Autodesk Inventor part; units mm, degrees
ref_plane "YZ Plane" through (0, 0, 0) normal (1, 0, 0) x (0, 1, 0)
ref_plane "XZ Plane" through (0, 0, 0) normal (0, 1, 0) x (-1, 0, 0)
ref_plane "XY Plane" through (0, 0, 0) normal (0, 0, 1) x (1, 0, 0)
sketch "Szkic1" plane through (0, 0, 0) normal (0, 1, 0) x (-1, 0, 0)
  line L0 (0, 0) -> (-15, 0)
  line L1 (0, 0) -> (15, 0)
  circle A0 centre (0, 0) radius 5
  circle A1 centre (15, 0) radius 2
  circle A2 centre (-15, 0) radius 2
  line L2 (-19, 7.5) -> (19, 7.5)
  line L3 (19, 7.5) -> (19, -7.5)
  line L4 (19, -7.5) -> (-19, -7.5)
  line L5 (-19, -7.5) -> (-19, 7.5)
  line L6 (-19, 7.5) -> (19, -7.5) construction
  line L7 (19, 7.5) -> (-19, -7.5) construction
  line L8 (0, 0) -> (15, 0)
  line L9 (6, 2.5) -> (9, 2.5)
  line L10 (9, 2.5) -> (9, -2.5)
  line L11 (9, -2.5) -> (6, -2.5)
  line L12 (6, -2.5) -> (6, 2.5)
  line L13 (6, 2.5) -> (9, -2.5) construction
  line L14 (9, 2.5) -> (6, -2.5) construction
  line L15 (-9, 2.5) -> (-6, 2.5)
  line L16 (-6, 2.5) -> (-6, -2.5)
  line L17 (-6, -2.5) -> (-9, -2.5)
  line L18 (-9, -2.5) -> (-9, 2.5)
  line L19 (-9, 2.5) -> (-6, -2.5) construction
  line L20 (-6, 2.5) -> (-9, -2.5) construction
  point P0 (7.5, 0)
  point P1 (-7.5, 0)
  point P2 (-5, 0)
  point P3 (5, 0)
  dimension "d0" = 15
  dimension "d1" = 15
  dimension "d2" = 10
  dimension "d3" = 4
  dimension "d4" = 4
  dimension "d5" = 38
  dimension "d6" = 15
  dimension "d7" = 3
  dimension "d8" = 5
  dimension "d9" = 3
  dimension "d10" = 5
extrude "Wyciągnięcie proste1" add sketch "Szkic1" along normal blind 1 contours L16 L17 L18 L0 | L0 L18 L15 L16 | L12 L9 L10 L1 | L1 L10 L11 L12 | L2 L3 L4 L5
extrude "Wyciągnięcie proste2" add sketch "Szkic1" along normal blind 30 contours L16 L17 L18 L0 | L0 L18 L15 L16
sketch "Szkic2" plane through (-6, 1, -2.5) normal (1, 0, 0) x (0, 0, -1)
  line L0 (0, 19) -> (-5, 19)
  line L1 (0, 19) -> (-2.12132, 16.87868)
  line L2 (0, 19) -> (3, 19) construction
  circle A0 centre (-2.12132, 16.87868) radius 1.5
  point P0 (-2.5, -1)
  dimension "d15" = 3
  dimension "d16" = 135
  dimension "d17" = 3
extrude "Wyciągnięcie proste3" [suppressed]
fillet "Zaokrąglenie1" radius 1 4 edges at (6, 15.5, -2.5) (9, 15.5, -2.5) (9, 15.5, 2.5) (6, 15.5, 2.5)
sketch "Szkic3" plane through (6, 1, 1.5) normal (-1, 0, 0) x (0, 0, 1)
  line L0 (-1.5, 27) -> (-1.5, 25)
  circle A0 centre (-1.5, 25) radius 1.5
  line L1 (-1.5, 25) -> (-1.5, 15)
  circle A1 centre (-1.5, 15) radius 1.5
  line L2 (-3, 29) -> (0, 29)
  point P0 (-1.5, -1)
  point P1 (0, 19)
  point P2 (-3, 19)
  point P3 (-1.5, 29)
  dimension "d21" = 2
  dimension "d22" = 3
  dimension "d23" = 10
  dimension "d24" = 3
  dimension "d28" = 2
sketch "Szkic3 outline for Wyciągnięcie proste4" plane through (6, 1, 1.5) normal (-1, 0, 0) x (0, 0, 1)
  circle A0 centre (-1.5, 25) radius 1.5
  circle A1 centre (-1.5, 15) radius 1.5
extrude "Wyciągnięcie proste4" add sketch "Szkic3 outline for Wyciągnięcie proste4" along normal blind 3 draft -3
fillet "Zaokrąglenie2" radius 0.6 8 edges at (-19, 0.5, 7.5) (-19, 0.5, -7.5) (-19, 1, 0) (0, 1, 7.5) (19, 1, 0) (19, 0.5, 7.5) (19, 0.5, -7.5) (0, 1, -7.5)
properties part number "sensor_holder" material "Tworzywo sztuczne ABS"
Check sheet for the modelled part. Datum: model origin and axes. Units: mm. A direction names the side the tool comes from. Round coordinates to 2 decimals unless told otherwise and drop trailing zeros. Order: outer loops, then holes, each group sorted by start corner. A loop starts at its lowest first (then second) coordinate and runs counter-clockwise, first axis right, second up. Notation, with made-up numbers: (5.5, -12.75) - (57.5, -12.75) arc R21 cw to (57.5, 11.25) - close; hole circle Ø2 at (18.25, 53.5). An arc over 180 degrees is marked (long way). Write item = value, one per line.
Q1. Section check A-A (x = -15). Record the boundary of the cut face in (y, z), and give its area (3 significant figures).
Computed:
outline = (0, -7.5) - (0.4, -7.5) arc R0.6 ccw to (1, -6.9) - (1, -2) - (0, -2) - close; (0, 2) - (1, 2) - (1, 6.9) arc R0.6 ccw to (0.4, 7.5) - (0, 7.5) - close
area = 10.8 mm^2
Q2. Section check C-C (y = 23.5). Record the boundary of the cut face in (x, z).
Computed:
outline = (6, -1.5) arc R1 ccw to (7, -2.5) - (8, -2.5) arc R1 ccw to (9, -1.5) - (9, 1.5) arc R1 ccw to (8, 2.5) - (7, 2.5) arc R1 ccw to (6, 1.5) - close
Q3. Section check B-B (z = 0). State how many separate pieces and enclosed holes the cut face has, and give its area (3 significant figures).
Computed:
separate_pieces = 4
enclosed_holes = 0
area = 124 mm^2
Q4. Thickness scan on line 1 along Z through (x, y) = (0, 0.5); line 2 along Z through (x, y) = (-15, 0.2); line 3 along Y through (x, z) = (-10.5, 5.25). Record the ranges inside material, lowest first.
Computed:
line_1 = -7.49 to -5, 5 to 7.49
line_2 = -7.5 to -2, 2 to 7.5
line_3 = 0 to 1
Q5. Section check D-D (x = 11). Record the boundary of the cut face in (y, z).
Computed:
outline = (0, -7.5) - (0.4, -7.5) arc R0.6 ccw to (1, -6.9) - (1, 6.9) arc R0.6 ccw to (0.4, 7.5) - (0, 7.5) - close
Q6. Go/stop test with flat-tipped pins: pin 1 (8 mm diameter, centred on x = 0, z = 0, fed in from +Y); pin 2 (6 mm diameter, centred on x = -11.5, z = 3.5, fed in from +Y); pin 3 (2 mm diameter, centred on y = 25.5, z = -0.5, fed in from -X). Record where each tip stops, or that it passes through.
Computed:
pin_1 = 27.4
pin_2 = 1
pin_3 = 3
Q7. Draft check along Z on faces 6 (the face through (6.301, 15.703, -2.215)), 7 (the face through (16.6, 0.5, 1.2)), 8 (the face through (6.285, 15.703, 2.199)), 9 (the face through (4.5, 0, 3.4)). Enter one of: pulls with the +Z half, pulls with the -Z half, needs draft (parallel to the pull), parting line crosses it, or undercut.
Computed:
face_6 = pulls with the -Z half
face_7 = undercut
face_8 = pulls with the +Z half
face_9 = needs draft
Q8. Tool access check on faces 1 (the face through (-13.4, 0.5, 1.2)), 2 (the face through (8.699, 15.703, 2.215)), 3 (the face through (7.5, 15.3, 2.5)), 4 (the face through (7.5, 15.3, -2.5)), 5 (the face through (8.715, 15.703, -2.199)). Record the directions out of +Z, -Z, +X, -X, +Y, -Y that give a thin tool (end or side, any length) a straight path to the whole face; none if there is none.
Computed:
face_1 = +Y, -Y
face_2 = +Z, +X, +Y
face_3 = +Z, +X, -X, +Y
face_4 = -Z, +X, -X, +Y
face_5 = -Z, +X, +Y
